Autodesk Inventor part; units mm, degrees
ref_plane "YZ Plane" through (0, 0, 0) normal (1, 0, 0) x (0, 1, 0)
ref_plane "XZ Plane" through (0, 0, 0) normal (0, 1, 0) x (-1, 0, 0)
ref_plane "XY Plane" through (0, 0, 0) normal (0, 0, 1) x (1, 0, 0)
sketch "Esquisse1" plane through (0, 0, 0) normal (1, 0, 0) x (0, 1, 0)
  line L0 (2.5227, 0) -> (-2.5227, 0)
  line L1 (0, 5) -> (75.5, 5)
  line L2 (76, 8.5) -> (76, 12)
  line L3 (76, 12) -> (76.5, 12.5)
  line L4 (76.5, 12.5) -> (106, 12.5)
  line L5 (0, 5) -> (0, 0)
  line L6 (0, 0) -> (109.25, 0)
  line L7 (106.5, 5) -> (106.5, 12)
  line L8 (106, 12.5) -> (106.5, 12)
  line L9 (76, 8.5) -> (75.5, 7.5)
  line L10 (75.5, 7.5) -> (75.5, 5)
  line L11 (109.25, 0) -> (109.25, 4.5)
  line L12 (109.25, 4.5) -> (108.75, 5)
  line L13 (108.75, 5) -> (106.5, 5)
  dimension "d2" = 0.5
  dimension "d3" = 0.5
  dimension "d6" = 10
  dimension "d7" = 76
  dimension "d8" = 25
  dimension "d9" = 0.5
  dimension "d10" = 0.5
  dimension "d11" = 30.5
  dimension "d13" = 1
  dimension "d14" = 0.5
  dimension "d15" = 17
  dimension "d23" = 0.5
  dimension "d24" = 0.5
  dimension "d25" = 10
  dimension "d26" = 2.75
revolve "Révolution1" add sketch "Esquisse1" angle 360 about axis through (0, 2.5227, 0) along (0, -1, 0)
thread "Filetage2"
chamfer "Chanfrein1" distance 0.5 angle 45 1 edges at (0, 0, -5)
sketch "Esquisse4" plane through (0, 109.25, 0) normal (0, 1, 0) x (1, 0, 0)
  circle A0 centre (0, 0) radius 4.5
  point P0 (0, 0)
hole "Perçage2" at (0, 109.25, 0) direction (0, -1, 0) diameter 4.917 depth 17.1 tip angle 118
equation "\"d3\" = d2"
equation "\"d10\" = d9"
equation "\"d24\" = d23"
properties part number "axe_rotation_principal"
Design review of the part built by this model. Coordinates are the model's own, in mm. A direction names the side the tool comes from. Coordinates: 2 decimals unless noted, no trailing zeros. Order: outer loops, then holes, each group sorted by start corner. A loop starts at its lowest first (then second) coordinate and runs counter-clockwise, first axis right, second up.
1) Wall thickness on line 1 along X through (y, z) = (96, 0); line 2 along Y through (x, z) = (4, 5): over which ranges is each line inside the solid? List them lowest first.
2) For faces 4 (the flat face through (-0.2, 106.5, 5.2)), 5 (the flat face through (-8.2, 76, -2.8)), 6 (the flat face through (0, 0, 0)), list the 3-axis set-ups (+Z, -Z, +X, -X, +Y, -Y) from which the entire face can be reached by the end or side of a thin tool; tool diameter is ignored.
3) Clearance check with flat-ended pins moving along their axes: pin 1 (12 mm diameter, centred on x = -5.5, y = 37.5, fed in from -Z); pin 2 (1.5 mm diameter, centred on x = 1, y = 61.5, fed in from +Z); pin 3 (12 mm diameter, centred on x = 8.5, y = 30.5, fed in from +Z). State where each tip first meets the part, or that it passes through.
4) Take a section at A-A, the plane y = 59. Give the boundary of the cut face in (x, z).
5) Mouldability with a two-part tool opening along Z and no side actions: class faces 1 (the flat face through (2, 109.25, 2)), 2 (the cylindrical face through (-0.738, 100.58, 2.345)), 3 (the cylindrical face through (4.88, 107.61, -1.08)) as +Z half, -Z half, draft (parallel to the pull), parting line (faces both ways), or undercut.
Returned:
1. line 1: x = -12.5 to -2.46, 2.46 to 12.5
1. line 2: y = 75.5 to 106.5
2. face 4: +Y
2. face 5: -Y
2. face 6: +Z, -Z, +X, -X, -Y
3. pin 1: stops at z = -5
3. pin 2: stops at z = 4.99
3. pin 3: stops at z = 4.33
4. outline: circle Ø10 at (0, 0)
5. face 1: draft
5. face 2: undercut
5. face 3: parting line
